Could you check a few things on this model? Use its own coordinates, in mm. A direction names the side the tool comes from. Coordinates: 2 decimals unless noted, no trailing zeros. Write each loop counter-clockwise with the first axis right and the second up, starting at its lowest first coordinate (ties: lowest second). Pieces come first, ordered by that corner, then holes. Notation, with made-up numbers: (-2.5, -5) - (55.5, -5) arc R32 ccw to (55.5, 31) - close; hole circle Ø7 at (26, 77.5). An arc over 180 degrees is marked (long way). Write item = value, one per line. Start each with the question number.
```python
from build123d import *

# Parameters (mm, degrees)
F0_W      = 12
F0_H      = 6.35
F1_DEPTH  = 4
F3_DEPTH  = 7
F4_W      = 12
F4_H      = 6.35
F5_DEPTH  = 4
F6_R      = 1.778
F7_DEPTH  = 25.4
F8_W      = 12
F8_H      = 5.35
F9_DEPTH  = 1
F10_W     = 12
F10_H     = 5.35
F11_DEPTH = 1
F12_F1_R  = 2.54
F12_F2_R  = 2.54


with BuildPart() as f1:
    # F0 (on Right) → F1 (new body)
    with BuildSketch(Plane.YZ):
        with Locations((6, 3.175)):
            Rectangle(F0_W, F0_H)
    extrude(amount=F1_DEPTH)

    # F2 (on face) → F3 (join)
    with BuildSketch(Plane.YZ.offset(4)):
        with BuildLine():
            ThreePointArc((10.2598245749, 1.38), (10.3587316459, 1.3427714117), (10.4085431086, 1.2495652174))
            ThreePointArc((10.4085431086, 1.2495652174), (10.4423882857, 1.091937846), (10.5011235955, 0.9417977528))
            ThreePointArc((10.5011235955, 0.9417977528), (11, 0.63), (11.4988764045, 0.9417977528))
            ThreePointArc((11.4988764045, 0.9417977528), (11.5576117143, 1.091937846), (11.5914568914, 1.2495652174))
            ThreePointArc((11.5914568914, 1.2495652174), (11.6412683541, 1.3427714117), (11.7401754251, 1.38))
            Line((11.7401754251, 1.38), (12, 1.38))
            Line((12, 1.38), (12, 6.35))
            Line((12, 6.35), (1, 6.35))
            Line((1, 6.35), (1, 2.38))
            ThreePointArc((1, 2.38), (1.2928932188, 1.6728932188), (2, 1.38))
            Line((2, 1.38), (2.2598245749, 1.38))
            ThreePointArc((2.2598245749, 1.38), (2.3587316459, 1.3427714117), (2.4085431086, 1.2495652174))
            ThreePointArc((2.4085431086, 1.2495652174), (2.4423882857, 1.091937846), (2.5011235955, 0.9417977528))
            ThreePointArc((2.5011235955, 0.9417977528), (3, 0.63), (3.4988764045, 0.9417977528))
            ThreePointArc((3.4988764045, 0.9417977528), (3.5576117143, 1.091937846), (3.5914568914, 1.2495652174))
            ThreePointArc((3.5914568914, 1.2495652174), (3.6412683541, 1.3427714117), (3.7401754251, 1.38))
            Line((3.7401754251, 1.38), (4, 1.38))
            Line((4, 1.38), (4.2598245749, 1.38))
            ThreePointArc((4.2598245749, 1.38), (4.3587316459, 1.3427714117), (4.4085431086, 1.2495652174))
            ThreePointArc((4.4085431086, 1.2495652174), (4.4423882857, 1.091937846), (4.5011235955, 0.9417977528))
            ThreePointArc((4.5011235955, 0.9417977528), (5, 0.63), (5.4988764045, 0.9417977528))
            ThreePointArc((5.4988764045, 0.9417977528), (5.5576117143, 1.091937846), (5.5914568914, 1.2495652174))
            ThreePointArc((5.5914568914, 1.2495652174), (5.6412683541, 1.3427714117), (5.7401754251, 1.38))
            Line((5.7401754251, 1.38), (6, 1.38))
            Line((6, 1.38), (6.2598245749, 1.38))
            ThreePointArc((6.2598245749, 1.38), (6.3587316459, 1.3427714117), (6.4085431086, 1.2495652174))
            ThreePointArc((6.4085431086, 1.2495652174), (6.4423882857, 1.091937846), (6.5011235955, 0.9417977528))
            ThreePointArc((6.5011235955, 0.9417977528), (7, 0.63), (7.4988764045, 0.9417977528))
            ThreePointArc((7.4988764045, 0.9417977528), (7.5576117143, 1.091937846), (7.5914568914, 1.2495652174))
            ThreePointArc((7.5914568914, 1.2495652174), (7.6412683541, 1.3427714117), (7.7401754251, 1.38))
            Line((7.7401754251, 1.38), (8, 1.38))
            Line((8, 1.38), (8.2598245749, 1.38))
            ThreePointArc((8.2598245749, 1.38), (8.3587316459, 1.3427714117), (8.4085431086, 1.2495652174))
            ThreePointArc((8.4085431086, 1.2495652174), (8.4423882857, 1.091937846), (8.5011235955, 0.9417977528))
            ThreePointArc((8.5011235955, 0.9417977528), (9, 0.63), (9.4988764045, 0.9417977528))
            ThreePointArc((9.4988764045, 0.9417977528), (9.5576117143, 1.091937846), (9.5914568914, 1.2495652174))
            ThreePointArc((9.5914568914, 1.2495652174), (9.6412683541, 1.3427714117), (9.7401754251, 1.38))
            Line((9.7401754251, 1.38), (10, 1.38))
            Line((10, 1.38), (10.2598245749, 1.38))
        make_face()
    extrude(amount=F3_DEPTH)

    # F4 (on face) → F5 (join)
    with BuildSketch(Plane.YZ.offset(11)):
        with Locations((6, 3.175)):
            Rectangle(F4_W, F4_H)
    extrude(amount=F5_DEPTH)

    # F6 (on face) → F7 (cut)
    with BuildSketch(Plane.XY.offset(6.35)):
        with Locations((2, 6)):
            Circle(F6_R)
        with Locations((13, 6)):
            Circle(F6_R)
    extrude(amount=-F7_DEPTH, mode=Mode.SUBTRACT)

    # F8 (on face) → F9 (join)
    with BuildSketch(Plane(origin=(0, 0, 0), x_dir=(0, -1, 0), z_dir=(-1, 0, 0))):
        with Locations((-6, 3.675)):
            Rectangle(F8_W, F8_H)
    extrude(amount=F9_DEPTH)

    # F10 (on face) → F11 (join)
    with BuildSketch(Plane.YZ.offset(15)):
        with Locations((6, 3.675)):
            Rectangle(F10_W, F10_H)
    extrude(amount=F11_DEPTH)

    # F12: fillet of radius 2.54 on 3 edges, made by hand

    # F12_f1
    f12_f1_edges = [f1.edges().sort_by_distance(p)[0] for p in [
        (1.5, 0, 6.35),
    ]]
    fillet(f12_f1_edges, radius=F12_F1_R)

    # F12_f2
    f12_f2_edges = [f1.edges().sort_by_distance(p)[0] for p in [
        (7.5, 12, 6.35),
    ]]
    fillet(f12_f2_edges, radius=F12_F2_R)


solid = f1.part
```
1) Which directions (+Z, -Z, +X, -X, +Y, -Y) give clear straight access to the entire face, cutting with the end or side of a thin tool? Please do faces 4 (the flat face through (15, 5.9, 0.5)), 5 (the cylindrical face through (7.451, 1.285, 1.681)), 6 (the flat face through (7, 1, 4)).
2) For P1, Ø2, axis at x = 8, z = 2.5, coming from the -Y side; P2, Ø3, axis at x = 13, y = 6, coming from the -Z side, each with a flat end and sliding along its axis, tell me the tip position at first contact or that it passes through.
3) If I drill on probe 1 along X at (y, z) = (0.75, 1.5); probe 2 along Y at (x, z) = (13, 2.5); probe 3 along X at (y, z) = (6.5, 5.25), over which ranges is the centre line in solid material (lowest first)? Write a range as [from, to].
4) Suppose I cut it at C-C on z = 3. Please give me the cut outline in (x, y), plus the area to 3 significant figures.
5) Thinking about a two-plate mould opening in X: for faces 1 (the flat face through (0.6, 4.6, 0)), 2 (the cylindrical face through (7.45, 10.99, 0.63)), 3 (the flat face through (-1, 6, 4)), which applies, +X half, -X half, draft (parallel to the pull), parting line (faces both ways), or undercut?
6) Suppose I cut it at B-B on x = 13. Please give me the cut outline in (y, z).
7) Suppose I cut it at A-A on y = 6. Please give me the cut outline in (x, z), plus the area to 3 significant figures.
8) Suppose I cut it at D-D on y = 11.25. Please give me the cut outline in (x, z), plus the area to 3 significant figures.
Reply:
q1.face_4 = -Z, +X, +Y, -Y
q1.face_5 = -Z, -Y
q1.face_6 = +Z, -Z, -Y
q2.P1 = 1
q2.P2 = through
q3.probe_1 = [-1, 4], [11, 16]
q3.probe_2 = [0, 4.22], [7.78, 12]
q3.probe_3 = [-1, 0.29], [3.71, 11.29], [14.71, 16]
q4.outline = (-1, 0) - (4, 0) - (4, 1) - (11, 1) - (11, 0) - (16, 0) - (16, 12) - (-1, 12) - close; hole circle Ø3.56 at (2, 6); hole circle Ø3.56 at (13, 6)
q4.area = 177 mm^2
q5.face_1 = draft
q5.face_2 = undercut
q5.face_3 = -X half
q6.outline = (0, 0) - (4.22, 0) - (4.22, 6.35) - (2.54, 6.35) arc R2.54 ccw to (0, 3.81) - close; (7.78, 0) - (12, 0) - (12, 3.81) arc R2.54 ccw to (9.46, 6.35) - (7.78, 6.35) - close
q7.outline = (-1, 1) - (0, 1) - (0, 0) - (0.22, 0) - (0.22, 6.35) - (-1, 6.35) - close; (3.78, 0) - (4, 0) - (4, 1.38) - (11, 1.38) - (11, 0) - (11.22, 0) - (11.22, 6.35) - (3.78, 6.35) - close; (14.78, 0) - (15, 0) - (15, 1) - (16, 1) - (16, 6.35) - (14.78, 6.35) - close
q7.area = 51.1 mm^2
q8.outline = (-1, 1) - (0, 1) - (0, 0) - (4, 0) - (4, 0.69) - (11, 0.69) - (11, 0) - (15, 0) - (15, 1) - (16, 1) - (16, 5.61) - (-1, 5.61) - close
q8.area = 88.6 mm^2
